```python
from build123d import *

# Parameters (mm, degrees)
SKETCH1_R               = 5.35
BOSS_EXTRUDE2_DEPTH     = 7
BOSS_EXTRUDE3_START     = 8
SKETCH3_R               = 5.35
BOSS_EXTRUDE3_DEPTH     = 8
BOSS_EXTRUDE4_DEPTH     = 3
FILLET1_R               = 1
CHAMFER1_SIZE           = 10
CHAMFER2_SIZE           = 5
CUT_EXTRUDE1_DEPTH      = 67.560662475
CUT_EXTRUDE1_DEPTH_BACK = 67.560662475
SKETCH5_W               = 33.474956737
SKETCH5_H               = 3.5
SKETCH5_H_2             = 8
CHAMFER3_SIZE           = 7
SKETCH6_R               = 11
BOSS_EXTRUDE5_DEPTH     = 5
SKETCH8_W               = 3
SKETCH8_H               = 7.519820499
SKETCH8_H_2             = 11.230179501
CUT_EXTRUDE2_DEPTH      = 5


# Some blends are built 0.0001 mm under size
with BuildPart() as part:
    # Sketch1 → Boss-Extrude2 (new body)
    with BuildSketch(Plane.XY):
        Polygon((-19.503784034, -20), (19.503784034, -20), (19.503784034, -18.25), (62.978740771, -18.25), (62.978740771, 13), (19.503784034, 13), (19.503784034, 20), (-19.503784034, 20), align=None)
        Circle(SKETCH1_R, mode=Mode.SUBTRACT)
    extrude(amount=-BOSS_EXTRUDE2_DEPTH)

    # Sketch3 → Boss-Extrude3 (add)
    with BuildSketch(Plane.XY.offset(BOSS_EXTRUDE3_START)):
        with BuildLine():
            Line((7.668115805, 5.35), (62.978740771, 5.35))
            Line((62.978740771, 5.35), (62.978740771, 9.35))
            Line((62.978740771, 9.35), (0, 9.35))
            ThreePointArc((0, 9.35), (-9.35, 0), (0, -9.35))
            Line((0, -9.35), (62.978740771, -9.35))
            Line((62.978740771, -9.35), (62.978740771, -5.35))
            Line((62.978740771, -5.35), (7.668115805, -5.35))
            ThreePointArc((7.668115805, -5.35), (9.35, 0), (7.668115805, 5.35))
        make_face()
        Circle(SKETCH3_R, mode=Mode.SUBTRACT)
    extrude(amount=-BOSS_EXTRUDE3_DEPTH)

    # Sketch4 → Boss-Extrude4 (add)
    with BuildSketch(Plane.XY):
        with BuildLine():
            Line((0, -18.25), (62.978740771, -18.25))
            Line((62.978740771, -18.25), (62.978740771, -16.25))
            Line((62.978740771, -16.25), (8.306623863, -16.25))
            Line((8.306623863, -16.25), (0, -16.25))
            ThreePointArc((0, -16.25), (-16.25, 0), (0, 16.25))
            Line((0, 16.25), (0, 18.25))
            ThreePointArc((0, 18.25), (-18.25, 0), (0, -18.25))
        make_face()
    extrude(amount=BOSS_EXTRUDE4_DEPTH)

    # Fillet1
    fillet1_edges = [part.edges().sort_by_distance(p)[0] for p in [
        (0, 16.25, 1.5),
        (0, 18.25, 1.5),
    ]]
    fillet(fillet1_edges, radius=FILLET1_R - 0.0001)  # a hair under: the kernel refuses the full size

    # Chamfer1
    # the kernel refuses this chamfer: 10 mm, written as the material it takes off along each edge
    with BuildSketch(Plane(origin=(19.503784034, -20, 25.71682988), x_dir=(0.027495876610586317, 0.9996219169112968, 0), z_dir=(0, 0, -1))) as chamfer1_piece_1_section:
        Polygon((CHAMFER1_SIZE * 0.999621916911, -CHAMFER1_SIZE * 0.0274958766106), (-CHAMFER1_SIZE * 0.0274958766106, -CHAMFER1_SIZE * 0.999621916911), (0, 0), align=None)
    chamfer1_piece_1 = extrude(amount=58.433659759, mode=Mode.PRIVATE)
    chamfer1_piece_1 = split(chamfer1_piece_1, bisect_by=Plane(origin=(14.814200223, -18.25, -3.5), z_dir=(0, -1, 0)), keep=Keep.TOP, mode=Mode.PRIVATE)
    add(chamfer1_piece_1, mode=Mode.SUBTRACT)

    # Chamfer2
    chamfer2_edges = [part.edges().sort_by_distance(p)[0] for p in [
        (-19.503784034, -20, -3.5),
        (-19.503784034, 20, -3.5),
    ]]
    chamfer(chamfer2_edges, length=CHAMFER2_SIZE)

    # Sketch5 → Cut-Extrude1 (cut, two sides: drawn at the far end of the back side and taken through both)
    with BuildSketch(Plane.XY.offset(-CUT_EXTRUDE1_DEPTH_BACK)):
        with Locations((36.241262403, 3.6)):
            Rectangle(SKETCH5_W, SKETCH5_H)
        with Locations((36.241262403, -7.15)):
            Rectangle(SKETCH5_W, SKETCH5_H_2)
    extrude(amount=CUT_EXTRUDE1_DEPTH + CUT_EXTRUDE1_DEPTH_BACK, mode=Mode.SUBTRACT)

    # Chamfer3
    chamfer3_edges = [part.edges().sort_by_distance(p)[0] for p in [
        (19.503784034, 20, -3.5),
    ]]
    chamfer(chamfer3_edges, length=CHAMFER3_SIZE - 0.0001)  # a hair under: the kernel refuses the full size


with BuildPart() as body_2:
    # Mirror9: mirrored copy
    add(part.part.mirror(Plane.XY.offset(-10)))

    # Sketch6 → Boss-Extrude5 (add)
    with BuildSketch(Plane.XY.offset(-13)):
        Circle(SKETCH6_R)
    extrude(amount=BOSS_EXTRUDE5_DEPTH)

    # Sketch8 → Cut-Extrude2 (cut)
    with BuildSketch(Plane(origin=(62.978740771, 0, 0), x_dir=(0, 0, -1), z_dir=(1, 0, 0))):
        with Locations((16.5, 6.240089751)):
            Rectangle(SKETCH8_W, SKETCH8_H)
        with Locations((16.5, -9.13491025)):
            Rectangle(SKETCH8_W, SKETCH8_H_2)
    extrude(amount=-CUT_EXTRUDE2_DEPTH, mode=Mode.SUBTRACT)


solid = body_2.part
```
CAD build for the part. Positions are in the model's coordinates, mm. A direction names the side the tool comes from. Round coordinates to 2 decimals unless told otherwise and drop trailing zeros. Loops run counter-clockwise (first coordinate to the right, second up) from the corner with the lowest first, then second, coordinate; pieces in that order, holes last. Notation, with made-up numbers: M -24.5,21 L 34.5,21 A29 cw 34.5,45 Z; hole C 37.25,61.5 d3. An arc over 180 degrees is marked long. Return JSON: item names as keys, results as strings. Group by question number.
(1) Mould opens along Z. For faces 4 (the flat face through (9, -10, -20)), 5 (the flat face through (21, 0, -13)), 6 (the flat face through (61, -9, -18)), 7 (the flat face through (38, -18.25, -18)) say: +Z half, -Z half, draft (parallel to the pull), parting line (faces both ways), or undercut.
(2) Saw through at C-C, the plane z = -19. Give the number of separate pieces and of enclosed holes in the cut face, and give its area (3 significant figures).
(3) Saw through at A-A, the plane x = 49.5. List the corners of the cut face in (y, z).
(4) Drop flat-ended pins along their axis: P1, Ø4, axis at x = 37.5, y = -13.5, coming from the +Z side; P2, Ø6, axis at x = 22, y = -13, coming from the -Z side; P3, Ø10, axis at x = 29.5, z = -20.5, coming from the -Y side; P4, Ø8, axis at y = -11, z = -10, coming from the -X side. Give the stop position or say it passes through.
(5) Saw through at D-D, the plane y = 0. List the corners of the cut face in (x, z), and give its area (3 significant figures).
(6) Tool access for faces 1 (the cylindrical face through (-18.25, -0.14, -21.48)), 2 (the flat face through (52.979, 4, -16)), 3 (the flat face through (57.979, -9, -16)): list every direction of +Z, -Z, +X, -X, +Y, -Y with a clear straight run to the whole face (end or side of a thin tool).
(7) Wall check: probe 1 along Y at (x, z) = (33, -19.75); probe 2 along Y at (x, z) = (0, -19.5); probe 3 along X at (y, z) = (-10.5, -15.5). Give the ranges that are in metal, low to high. Write a range as [from, to].
(8) Saw through at B-B, the plane z = -25.75. List the corners of the cut face in (x, y), and give its area (3 significant figures).
Answer list:
{
 "1": {"face 4": "-Z half", "face 5": "+Z half", "face 6": "undercut", "face 7": "draft"},
 "2": {"separate pieces": "1", "enclosed holes": "3", "area": "2,380 mm2"},
 "3": {"outline": "M -18.25,-23 L -16.25,-23 L -16.25,-20 L -11.15,-20 L -11.15,-13 L -18.25,-13 Z; M -3.15,-20 L 1.85,-20 L 1.85,-13 L -3.15,-13 Z; M 5.35,-28 L 9.35,-28 L 9.35,-20 L 13,-20 L 13,-13 L 5.35,-13 Z"},
 "4": {"P1": "z = -13", "P2": "z = -20", "P3": "y = -18.25", "P4": "x = -19.5"},
 "5": {"outline": "M -19.5,-20 L -18.25,-20 L -18.25,-23 L -16.25,-23 L -16.25,-20 L -9.35,-20 L -9.35,-28 L -5.35,-28 L -5.35,-13 L 5.35,-13 L 5.35,-28 L 9.35,-28 L 9.35,-20 L 62.98,-20 L 62.98,-13 L 11,-13 L 11,-8 L -11,-8 L -11,-13 L -19.5,-13 Z", "area": "682 mm2"},
 "6": {"face 1": "-Z, -X", "face 2": "+Z, -Z", "face 3": "+X"},
 "7": {"probe 1": "[-18.25, -11.15], [-3.15, 1.85], [5.35, 13]", "probe 2": "[-20, -5.35], [5.35, 20]", "probe 3": "[-19.5, 19.5], [52.98, 57.98]"},
 "8": {"outline": "M 0,-9.35 L 19.5,-9.35 L 19.5,-5.35 L 7.67,-5.35 A9.35 ccw 7.67,5.35 L 62.98,5.35 L 62.98,9.35 L 0,9.35 A9.35 ccw Z; M 52.98,-9.35 L 62.98,-9.35 L 62.98,-5.35 L 52.98,-5.35 Z; hole C 0,0 d10.7", "area": "512 mm2"}
}
